Can you work these out from the drawing? Everything is in mm from the part's minimum corner. A direction names the side the tool comes from. Give positions to 0.01 mm unless a question says otherwise; leave off trailing zeros. Write each loop counter-clockwise with the first axis right and the second up, starting at its lowest first coordinate (ties: lowest second). Pieces come first, ordered by that corner, then holes. Notation, with made-up numbers: (62, -9.75) - (114, -9.75) arc R20 ccw to (114, 28.25) - close; hole circle Ø4 at (42, -27.75). An arc over 180 degrees is marked (long way). Answer in a Markdown table with one row per item.
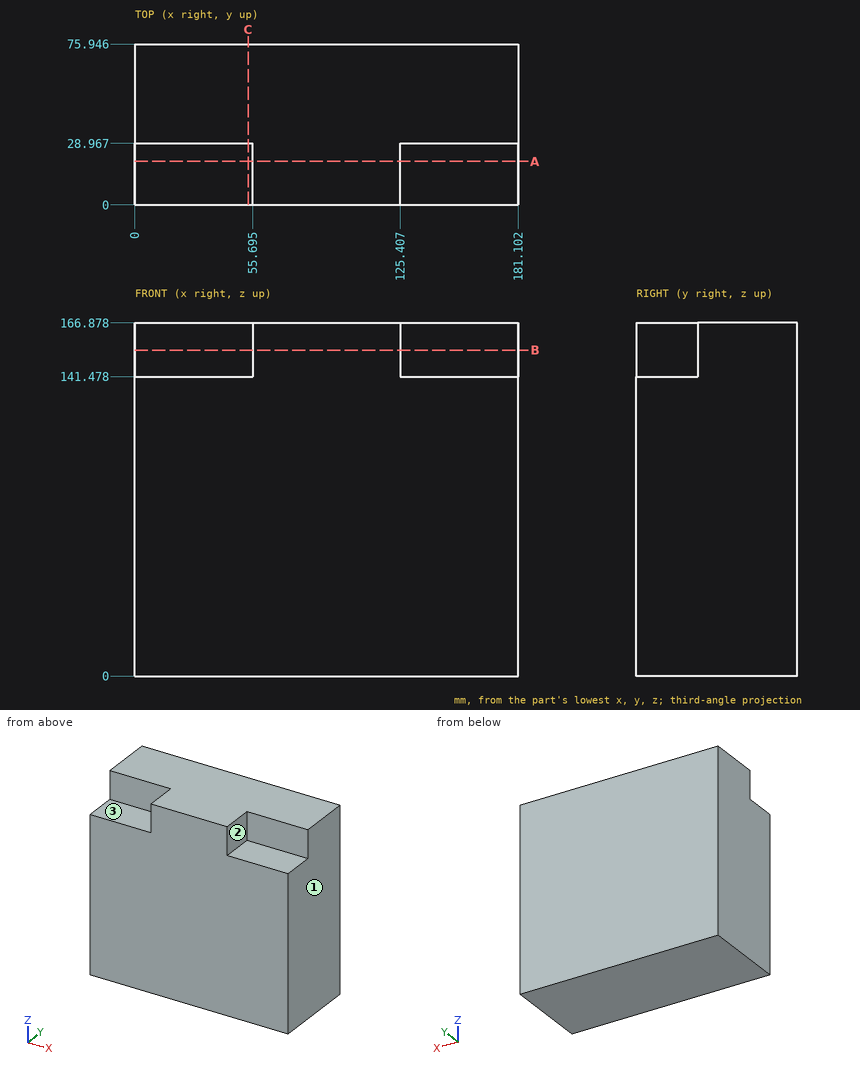
1) Imagine slicing it at A-A (y = 20.5). List the corners of the cut face in (x, z) for me (1 decimal).
Check values:
| item | result |
|---|---|
| outline | (0, 0) - (181.1, 0) - (181.1, 141.5) - (125.4, 141.5) - (125.4, 166.9) - (55.7, 166.9) - (55.7, 141.5) - (0, 141.5) - close |
2) Will these pins go through, and if not, where does the flat tip stop? P1, Ø20.5, axis at y = 13.5, z = 152, coming from the -X side (3 decimals); P2, Ø20.5, axis at x = 25.5, z = 154, coming from the -Y side; P3, Ø8.5, axis at x = 154, y = 13.5, coming from the +Z side.
Check values:
| item | result |
|---|---|
| P1 | stops at x = 55.695 |
| P2 | stops at y = 28.97 |
| P3 | stops at z = 141.48 |
3) If I drill on line 1 (Y direction, x = 29.5, z = 153.5); line 2 (X direction, y = 25, z = 148.5) (1 decimal); line 3 (Z direction, x = 165, y = 14), over which ranges is the centre line in solid material (lowest first)?
Check values:
| item | result |
|---|---|
| line 1 | y = 28.97 to 75.95 |
| line 2 | x = 55.7 to 125.4 |
| line 3 | z = 0 to 141.48 |
4) On a 3-axis mill with a long thin cutter (end or side, diameter ignored), from which of +Z, -Z, +X, -X, +Y, -Y can I reach the whole of each face in a straight line? I mean the marked faces 1, 2 and 3. Say none if no direction works.
Check values:
| item | result |
|---|---|
| face 1 | +Z, -Z, +X, +Y, -Y |
| face 2 | +Z, +X, -Y |
| face 3 | +Z, -X, -Y |
5) Imagine slicing it at C-C (x = 53.5). List the corners of the cut face in (y, z) for me, then the cut area to 3 significant figures.
Check values:
| item | result |
|---|---|
| outline | (0, 0) - (75.95, 0) - (75.95, 166.88) - (28.97, 166.88) - (28.97, 141.48) - (0, 141.48) - close |
| area | 11,900 mm2 |
6) Imagine slicing it at B-B (z = 154). List the corners of the cut face in (x, y) for me (1 decimal).
Check values:
| item | result |
|---|---|
| outline | (0, 29) - (55.7, 29) - (55.7, 0) - (125.4, 0) - (125.4, 29) - (181.1, 29) - (181.1, 75.9) - (0, 75.9) - close |
